Work out the finished part from the listing and answer in its coordinate system (mm). Round coordinates to 2 decimals unless told otherwise and drop trailing zeros. Write each loop counter-clockwise with the first axis right and the second up, starting at its lowest first coordinate (ties: lowest second). Pieces come first, ordered by that corner, then holes.
1. Find section B-B (x = -7). Write down the section's boundary in (y, z), and give its area (3 significant figures).
2. Flat-ended cylindrical pins translate along their axes: pin 1 Ø1.5 at (x, z) = (-25.5, 2.5) entering from +Y; pin 2 Ø1.5 at (x, z) = (-77, 3) entering from -Y. Find the tip coordinate at first contact, or state that the pin passes through.
3. Straight lines are drawn through the part: probe 1 along Y at (x, z) = (-61.35, 3.6); probe 2 along Y at (x, z) = (-18, 0.45); probe 3 along X at (y, z) = (8.5, 3.05). For each, find the intervals that lie inside material, in ascending order.
4. Find section D-D (y = 34.5). Write down the section's boundary in (x, z).
5. Find section C-C (x = 40.3). Write down the section's boundary in (y, z), and give its area (3 significant figures).
6. Find section A-A (y = 13.5). Write down the section's boundary in (x, z).
```python
from build123d import *

# Parameters (mm, degrees)
SKETCH1_W           = 135
SKETCH1_H           = 86
BOSS_EXTRUDE1_DEPTH = 5
SKETCH2_W           = 35.2
SKETCH2_H           = 5.1
CUT_EXTRUDE1_DEPTH  = 5
SKETCH3_W           = 25
SKETCH3_H           = 17
BOSS_EXTRUDE2_DEPTH = 5
SKETCH4_W           = 107.1
SKETCH4_H           = 68.6
CUT_EXTRUDE2_DEPTH  = 5
SKETCH5_R           = 2
CUT_EXTRUDE3_DEPTH  = 10
SKETCH6_R           = 4
SKETCH6_R_2         = 2
BOSS_EXTRUDE3_DEPTH = 5
SKETCH7_R           = 2
CUT_EXTRUDE4_DEPTH  = 5


with BuildPart() as part:
    # Sketch1 → Boss-Extrude1 (new body)
    with BuildSketch(Plane.XY):
        Rectangle(SKETCH1_W, SKETCH1_H)
    extrude(amount=BOSS_EXTRUDE1_DEPTH)

    # Sketch2 → Cut-Extrude1 (cut)
    with BuildSketch(Plane(origin=(0, 0, 0), x_dir=(-1, 0, 0), z_dir=(0, 0, -1))):
        with Locations((0.1, 40.45)):
            Rectangle(SKETCH2_W, SKETCH2_H)
    extrude(amount=-CUT_EXTRUDE1_DEPTH, mode=Mode.SUBTRACT)

    # Sketch3 → Boss-Extrude2 (add)
    with BuildSketch(Plane(origin=(0, 0, 0), x_dir=(-1, 0, 0), z_dir=(0, 0, -1))):
        with Locations((80, -28.5)):
            Rectangle(SKETCH3_W, SKETCH3_H)
        with Locations((-80, -28.5)):
            Rectangle(SKETCH3_W, SKETCH3_H)
    extrude(amount=-BOSS_EXTRUDE2_DEPTH)

    # Sketch4 → Cut-Extrude2 (cut)
    with BuildSketch(Plane(origin=(0, 0, 0), x_dir=(-1, 0, 0), z_dir=(0, 0, -1))):
        with Locations((0.2, -2.1)):
            Rectangle(SKETCH4_W, SKETCH4_H)
    extrude(amount=-CUT_EXTRUDE2_DEPTH, mode=Mode.SUBTRACT)

    # Sketch5 → Cut-Extrude3 (cut)
    with BuildSketch(Plane(origin=(0, 0, 0), x_dir=(-1, 0, 0), z_dir=(0, 0, -1))):
        with Locations((-40.3, 40.5)):
            Circle(SKETCH5_R)
        with Locations((-80.4, -28.5)):
            Circle(SKETCH5_R)
        with Locations((80.3, -28.5)):
            Circle(SKETCH5_R)
        with Locations((40.5, 40.5)):
            Circle(SKETCH5_R)
    extrude(amount=-CUT_EXTRUDE3_DEPTH, mode=Mode.SUBTRACT)

    # Sketch6 → Boss-Extrude3 (add)
    with BuildSketch(Plane(origin=(0, 0, 0), x_dir=(-1, 0, 0), z_dir=(0, 0, -1))):
        with Locations((40.5, 40.5)):
            Circle(SKETCH6_R)
        with Locations((40.5, 40.5)):
            Circle(SKETCH6_R_2, mode=Mode.SUBTRACT)
        with Locations((-40.3, 40.5)):
            Circle(SKETCH6_R)
        with Locations((-40.3, 40.5)):
            Circle(SKETCH6_R_2, mode=Mode.SUBTRACT)
    extrude(amount=-BOSS_EXTRUDE3_DEPTH)

    # Sketch7 → Cut-Extrude4 (cut)
    with BuildSketch(Plane(origin=(0, 0, 0), x_dir=(-1, 0, 0), z_dir=(0, 0, -1))):
        with Locations((61.35, -38.7)):
            Circle(SKETCH7_R)
        with Locations((-61.35, -38.7)):
            Circle(SKETCH7_R)
        with Locations((-61.35, 34.5)):
            Circle(SKETCH7_R)
        with Locations((61.35, 34.5)):
            Circle(SKETCH7_R)
    extrude(amount=-CUT_EXTRUDE4_DEPTH, mode=Mode.SUBTRACT)


solid = part.part
```
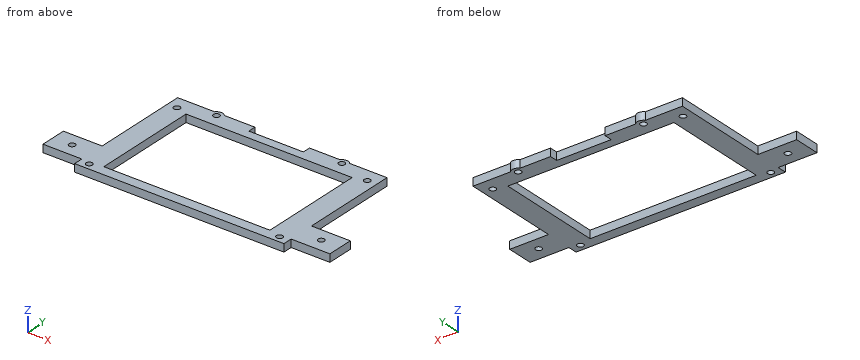
Worked answers:
1. outline: (-43, 0) - (-36.4, 0) - (-36.4, 5) - (-43, 5) - close; (32.2, 0) - (37.9, 0) - (37.9, 5) - (32.2, 5) - close
1. area: 61.5 mm2
2. pin 1: stops at y = 43
2. pin 2: stops at y = -37
3. probe 1: y = -43 to -40.7, -36.7 to 32.5, 36.5 to 43
3. probe 2: y = -43 to -36.4, 32.2 to 43
3. probe 3: x = -67.5 to -53.75, 53.35 to 67.5
4. outline: (-67.5, 0) - (-63.35, 0) - (-63.35, 5) - (-67.5, 5) - close; (-59.35, 0) - (59.35, 0) - (59.35, 5) - (-59.35, 5) - close; (63.35, 0) - (67.5, 0) - (67.5, 5) - (63.35, 5) - close
5. outline: (-43, 0) - (-36.4, 0) - (-36.4, 5) - (-43, 5) - close; (32.2, 0) - (38.5, 0) - (38.5, 5) - (32.2, 5) - close; (42.5, 0) - (44.5, 0) - (44.5, 5) - (42.5, 5) - close
5. area: 74.5 mm2
6. outline: (-67.5, 0) - (-53.75, 0) - (-53.75, 5) - (-67.5, 5) - close; (53.35, 0) - (67.5, 0) - (67.5, 5) - (53.35, 5) - close
